Geometry: see drawing. Coordinates: mm, zero at the bounding-box minimum. A direction names the side the tool comes from. Coordinates: 2 decimals unless noted, no trailing zeros. Write each loop counter-clockwise with the first axis right and the second up, starting at its lowest first coordinate (ties: lowest second). Pieces come first, ordered by that corner, then holes. Notation, with made-up numbers: M 9.5,52 L 62.5,52 A31 ccw 62.5,89 Z; hole C 1.5,50 d3. An arc over 180 degrees is marked long. Write item = value, one per line. Start each with the question number.
1. Pin query (flat end, axial travel): pin 1 Ø4 at (x, z) = (2.5, 9) entering from +Y; pin 2 Ø4 at (y, z) = (18, 1.5) entering from -X; pin 3 Ø2.5 at (x, y) = (12, 14.5) entering from -Z. Return the tip coordinate at first contact, or that it passes through.
2. Section query B-B (y = 2.75). Output: boundary loops of the cut face in (x, z).
3. Pull-direction query (X, two-part tool) for the marked faces 1, 2 and 3; classes: pulls with the +X half, pulls with the -X half, needs draft (parallel to the pull), parting line crosses it, or undercut.
4. Section query C-C (z = 11.5). Output: boundary loops of the cut face in (x, y).
5. Section query D-D (y = 12.5). Output: boundary loops of the cut face in (x, z).
6. Line query: line 1 along Z through (x, y) = (12.5, 4.5); line 2 along Y through (x, z) = (15.75, 11.5); line 3 along X through (y, z) = (2, 11.5). Output: solid intervals per line, ascending.
7. Section query A-A (x = 12.5). Output: boundary loops of the cut face in (y, z), then the cut area to 3 significant figures.
8. Access query for the marked faces 4, 5 and 6. Directions: +Z, -Z, +X, -X, +Y, -Y. A direction counts if a zero-diameter tool reaches every point of the face in a straight line with its end or side. Return the directions, or none.
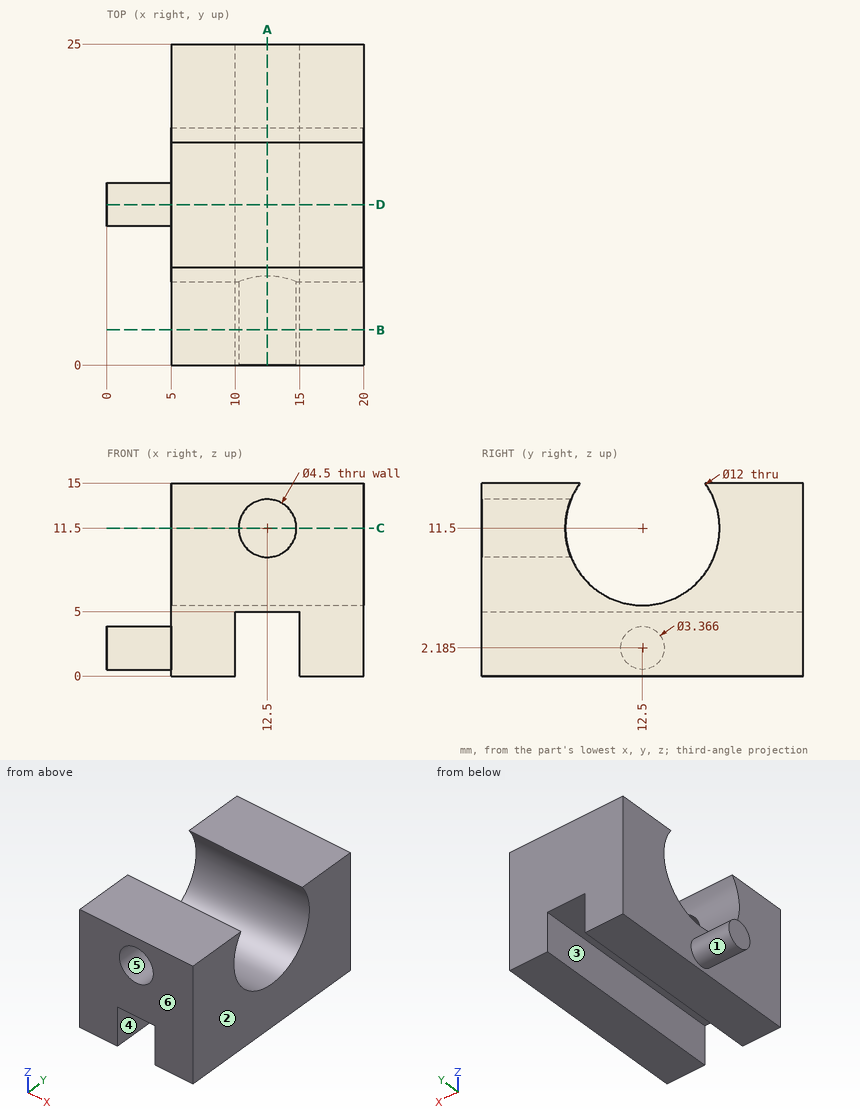
Results are:
q1.pin_1 = through
q1.pin_2 = 5
q1.pin_3 = 5
q2.outline = M 5,0 L 10,0 L 10,5 L 15,5 L 15,0 L 20,0 L 20,15 L 5,15 Z; hole C 12.5,11.5 d4.5
q3.face_1 = needs draft
q3.face_2 = pulls with the +X half
q3.face_3 = undercut
q4.outline = M 5,0 L 10.25,0 L 10.25,6.5 L 5,6.5 Z; M 5,18.5 L 20,18.5 L 20,25 L 5,25 Z; M 14.75,0 L 20,0 L 20,6.5 L 14.75,6.5 Z
q5.outline = M 0,0.5 L 5,0.5 L 5,0 L 10,0 L 10,5 L 15,5 L 15,0 L 20,0 L 20,5.5 L 5,5.5 L 5,3.87 L 0,3.87 Z
q6.line_1 = 5 to 9.25, 13.75 to 15
q6.line_2 = 0 to 6.5, 18.5 to 25
q6.line_3 = 5 to 10.25, 14.75 to 20
q7.outline = M 0,5 L 25,5 L 25,15 L 17.37,15 A6 cw long 6.94,9.25 L 0,9.25 Z; M 0,13.75 L 6.94,13.75 A6 cw 7.63,15 L 0,15 Z
q7.area = 124 mm^2
q8.face_4 = -Z, +Y, -Y
q8.face_5 = -Y
q8.face_6 = +Z, -Z, +X, -X, -Y
